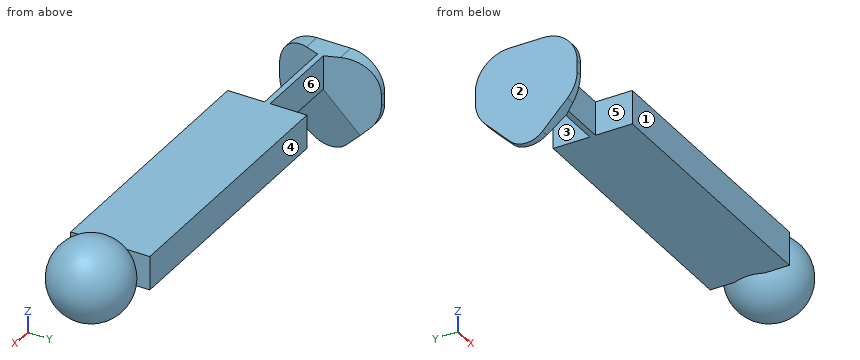
```python
from build123d import *

# Parameters (mm, degrees)
F2_W      = 23.6211707216
F2_H      = 3
F3_DEPTH  = 3.5
F6_DEPTH  = 2
F7_W      = 0.5
F7_H      = 3
F8_DEPTH  = 8
F12_DEPTH = 15
F14_DEPTH = 15


with BuildPart() as f1:
    # F0 (on Front) → F1 (revolve)
    with BuildSketch(Plane.XZ):
        with BuildLine():
            Line((-7, 0), (0, 0))
            ThreePointArc((0, 0), (-3.5, 3.5), (-7, 0))
        make_face()
    revolve(axis=Axis((-3.5, 0, 0), (1, 0, 0)))

    # F2 (on Front) → F3 (join, symmetric)
    with BuildSketch(Plane.XZ):
        with Locations((-18.1894146392, 0)):
            Rectangle(F2_W, F2_H)
    extrude(amount=F3_DEPTH, both=True)


with BuildPart() as f6:
    # F5 (on offset) → F6 (new body)
    with BuildSketch(Plane.YZ.offset(-40)):
        with BuildLine():
            ThreePointArc((4.5, -1.5), (3.6213203436, 0.6213203436), (1.5, 1.5))
            Line((1.5, 1.5), (-1.5, 1.5))
            ThreePointArc((-1.5, 1.5), (-3.6213203436, 0.6213203436), (-4.5, -1.5))
            Line((-4.5, -1.5), (-4.5, -2.5209097215))
            ThreePointArc((-4.5, -2.5209097215), (-4.2798610612, -3.6489046153), (-3.6517516798, -4.6113557764))
            Line((-3.6517516798, -4.6113557764), (-1.4345011199, -6.8936307033))
            ThreePointArc((-1.4345011199, -6.8936307033), (0, -7.5), (1.4345011199, -6.8936307033))
            Line((1.4345011199, -6.8936307033), (3.6517516798, -4.6113557764))
            ThreePointArc((3.6517516798, -4.6113557764), (4.2798610612, -3.6489046153), (4.5, -2.5209097215))
            Line((4.5, -2.5209097215), (4.5, -1.5))
        make_face()
    extrude(amount=F6_DEPTH)


with BuildPart() as f8:
    # F7 (on face) → F8 (new body, through all)
    with BuildSketch(Plane.YZ.offset(-38)):
        Rectangle(F7_W, F7_H)
    extrude(amount=F8_DEPTH)


with BuildPart() as f6_1:
    add(f6.part)

    # F9: union F8
    add(f8.part)


with BuildPart() as f1_1:
    add(f1.part)

    # F10: union F6
    add(f6_1.part)

    # F11 (on Top) → F12 (cut, symmetric)
    with BuildSketch(Plane.XY):
        Polygon((-39.5, 4.5), (-37.9991866648, 0.25), (-37.9909649491, 4.5), align=None)
        Polygon((-37.9909649491, -4.5), (-37.9991866648, -0.25), (-39.5, -4.5), align=None)
    extrude(amount=F12_DEPTH, both=True, mode=Mode.SUBTRACT)

    # F13 (on Front) → F14 (cut, symmetric)
    with BuildSketch(Plane.XZ):
        Polygon((-38, -7.5028174194), (-37.9915572703, -1.5), (-39.5, -7.5028174194), align=None)
    extrude(amount=F14_DEPTH, both=True, mode=Mode.SUBTRACT)


solid = f1_1.part
```
Read the model definition and answer for the solid it produces. Units are mm, in the model's axes. Face numbers are marked on the shaded views. A direction names the side the tool comes from. Give positions to 0.01 mm unless a question says otherwise; leave off trailing zeros. Write each loop counter-clockwise with the first axis right and the second up, starting at its lowest first coordinate (ties: lowest second). Pieces come first, ordered by that corner, then holes. Notation, with made-up numbers: (-23.5, -23) -> (35.5, -23) arc R19 ccw to (35.5, -6) -> close; hole circle Ø6 at (-6.75, 73.5). An arc over 180 degrees is marked (long way). Answer as a JSON object with one key per item and string values.
1) A tool of negligible diameter and unlimited length cuts with its end or side. For the marked faces 4, 5 and 6, from which of +Z, -Z, +X, -X, +Y, -Y can it reach the whole face along a straight path? Write none if from no direction.
Findings below:
{"face 4": "+Z, -Z, +X, +Y", "face 5": "+Z, -Z, -Y", "face 6": "+Z, -Z, +Y"}
2) Flat-ended cylindrical pins translate along their axes: pin 1 Ø5 at (x, z) = (-31, -3) entering from +Y; pin 2 Ø1.1 at (y, z) = (-3, -0.5) entering from +X; pin 3 Ø0.9 at (x, z) = (-35, 0) entering from -Y. Find the tip coordinate at first contact, or state that the pin passes through.
Findings below:
{"pin 1": "stops at y = 3.5", "pin 2": "stops at x = -1.04", "pin 3": "stops at y = -0.25"}
3) Section B-B on z = -3 is taken. Write down the section's boundary in (x, y), then the cut area to 3 significant figures.
Findings below:
{"outline": "(-40, -4.46) -> (-39.49, -4.46) -> (-38.37, -1.3) -> (-38.37, 1.3) -> (-39.49, 4.46) -> (-40, 4.46) -> close; circle Ø3.61 at (-3.5, 0)", "area": "21.2 mm^2"}
4) Straight lines are drawn through the part: probe 1 along X at (y, z) = (-2.5, 0.25); probe 2 along Z at (x, y) = (-22, 1.75); probe 3 along Y at (x, z) = (-28, 0). For each, find the intervals that lie inside material, in ascending order. Write a range as from..to.
Findings below:
{"probe 1": "x = -40..-38.79, -30..-6.38, -5.94..-1.06", "probe 2": "z = -1.5..1.5", "probe 3": "y = -3.5..3.5"}
5) Section A-A on y = 2 is taken. Write down the section's boundary in (x, z), then the cut area to 3 significant figures.
Findings below:
{"outline": "(-40, -6.31) -> (-39.2, -6.31) -> (-38.62, -3.99) -> (-38.62, 1.46) -> (-40, 1.46) -> close; (-30, -1.5) -> (-6.38, -1.5) -> (-6.38, 1.5) -> (-30, 1.5) -> close; circle Ø5.74 at (-3.5, 0)", "area": "107 mm^2"}
6) Section C-C on x = -36 is taken. Write down the section's boundary in (y, z), then the cut area to 3 significant figures.
Findings below:
{"outline": "(-0.25, -1.5) -> (0.25, -1.5) -> (0.25, 1.5) -> (-0.25, 1.5) -> close", "area": "1.50 mm^2"}
7) For a pull along X with two mould halves and no side action, classify the marked faces 1, 2 and 3 as pulls with the +X half, pulls with the -X half, needs draft (parallel to the pull), parting line crosses it, or undercut.
Findings below:
{"face 1": "needs draft", "face 2": "pulls with the -X half", "face 3": "undercut"}
